CAD build for the part. Positions are in the model's coordinates, mm. Round coordinates to 2 decimals unless told otherwise and drop trailing zeros. Loops run counter-clockwise (first coordinate to the right, second up) from the corner with the lowest first, then second, coordinate; pieces in that order, holes last. Notation, with made-up numbers: (-9, -35) -> (4, -35) arc R13 cw to (4, -28) -> close; hole circle Ø7 at (-35.75, 81). An arc over 180 degrees is marked (long way). Answer as CSV lines item,"result".
```python
from build123d import *

# Parameters (mm, degrees)
BOSS_EXTRUDE1_DEPTH = 21
SKETCH2_R           = 9
CUT_EXTRUDE1_DEPTH  = 40


with BuildPart() as part:
    # Sketch1 → Boss-Extrude1 (new body, symmetric)
    with BuildSketch(Plane.XY):
        Polygon((0, 0), (-60, 0), (-60, 30), (-15, 50), (0, 50), align=None)
    extrude(amount=BOSS_EXTRUDE1_DEPTH, both=True)

    # Sketch2 → Cut-Extrude1 (cut)
    with BuildSketch(Plane(origin=(0, 0, 0), x_dir=(0, 0, -1), z_dir=(1, 0, 0))):
        with Locations((0, 25)):
            Circle(SKETCH2_R)
    extrude(amount=-CUT_EXTRUDE1_DEPTH, mode=Mode.SUBTRACT)


solid = part.part
```
Q1. Slice it at C-C, the plane y = 25. Give the cut face in (x, z).
Results:
outline,"(-60, -21) -> (0, -21) -> (0, -9) -> (-40, -9) -> (-40, 9) -> (0, 9) -> (0, 21) -> (-60, 21) -> close"
Q2. Slice it at B-B, the plane x = -10. Give the cut face in (y, z), and give its area (3 significant figures).
Results:
outline,"(0, -21) -> (50, -21) -> (50, 21) -> (0, 21) -> close; hole circle Ø18 at (25, 0)"
area,"1,850 mm2"
Q3. Two-plate mould, pull along Z, no slides. Class faces 1 (the flat face through (-40, 25, 0)), 2 (the flat face through (-8, 50, 0)), 3 (the cylindrical face through (-19.72, 32.59, -4.84)), 4 (the flat face through (-30, 20, 21)): pulls with the +Z half, pulls with the -Z half, needs draft (parallel to the pull), parting line crosses it, or undercut.
Results:
face 1,"undercut"
face 2,"needs draft"
face 3,"undercut"
face 4,"pulls with the +Z half"
Q4. Drop flat-ended pins along their axis: pin 1 Ø3 at (x, z) = (-26, 15) entering from +Y; pin 2 Ø2 at (x, z) = (-23, 1) entering from +Y. Give the stop position or say it passes through.
Results:
pin 1,"y = 45.78"
pin 2,"y = 46.89"
Q5. Slice it at D-D, the plane z = -18. Give the cut face in (x, y).
Results:
outline,"(-60, 0) -> (0, 0) -> (0, 50) -> (-15, 50) -> (-60, 30) -> close"
Q6. Slice it at A-A, the plane z = 0. Give the cut face in (x, y), and give its area (3 significant figures).
Results:
outline,"(-60, 0) -> (0, 0) -> (0, 16) -> (-40, 16) -> (-40, 34) -> (0, 34) -> (0, 50) -> (-15, 50) -> (-60, 30) -> close"
area,"1,830 mm2"
Q7. Probe L1, parallel to Y at x = -7.5, z = 0; L2, parallel to Z at x = -27.5, y = 24.5; L3, parallel to Y at x = -22.5, z = 5. List the from-to ranges inside material, lowest first. Write a range as [from, to].
Results:
L1,"[0, 16], [34, 50]"
L2,"[-21, -8.99], [8.99, 21]"
L3,"[0, 17.52], [32.48, 46.67]"
